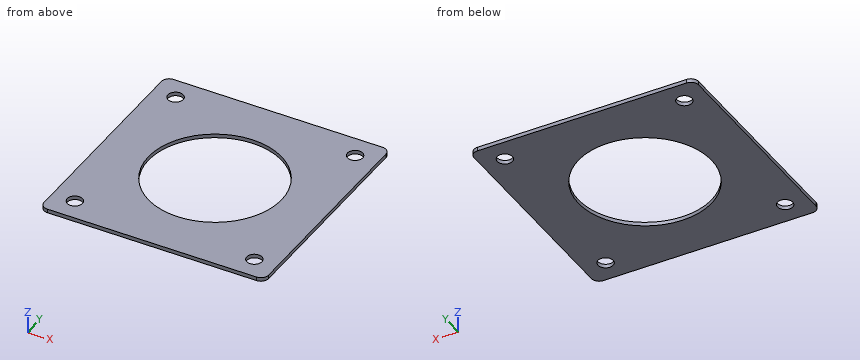
Autodesk Inventor part; units mm, degrees
ref_plane "YZ Plane" through (0, 0, 0) normal (1, 0, 0) x (0, 1, 0)
ref_plane "XZ Plane" through (0, 0, 0) normal (0, 1, 0) x (-1, 0, 0)
ref_plane "XY Plane" through (0, 0, 0) normal (0, 0, 1) x (1, 0, 0)
sketch "Sketch1" plane through (0, 0, 0) normal (0, 0, 1) x (1, 0, 0)
  line L0 (0, 0) -> (59, 0)
  line L1 (59, 0) -> (59, 59)
  line L2 (59, 59) -> (0, 59)
  line L3 (0, 59) -> (0, 0)
  dimension "d0" = 59
  dimension "d1" = 59
extrude "Extrusion1" add sketch "Sketch1" along normal blind 1
sketch "Sketch2" plane through (0, 0, 1) normal (0, 0, 1) x (1, 0, 0)
  circle A0 centre (29.5, 29.5) radius 17.5
  line L0 (59, 59) -> (0, 59)
  line L1 (0, 59) -> (0, 0)
  point P0 (29.5, 59)
  point P1 (0, 29.5)
  dimension "d4" = 35
extrude "Extrusion2" cut sketch "Sketch2" against normal through all
sketch "Sketch3" plane through (0, 0, 1) normal (0, 0, 1) x (1, 0, 0)
  line L0 (5.9, 5.9) -> (53.1, 5.9) construction
  line L1 (53.1, 5.9) -> (53.1, 53.1) construction
  line L2 (53.1, 53.1) -> (5.9, 53.1) construction
  line L3 (5.9, 53.1) -> (5.9, 5.9) construction
  line L4 (59, 59) -> (0, 59) construction
  line L5 (0, 59) -> (0, 0) construction
  circle A0 centre (5.9, 53.1) radius 2
  circle A1 centre (53.1, 53.1) radius 2
  circle A2 centre (53.1, 5.9) radius 2
  circle A3 centre (5.9, 5.9) radius 2
  point P0 (29.5, 53.1)
  point P1 (29.5, 59)
  point P2 (53.1, 29.5)
  point P3 (0, 29.5)
  dimension "d7" = 47.2
  dimension "d8" = 47.2
  dimension "d9" = 4
  dimension "d10" = 4
  dimension "d11" = 4
  dimension "d12" = 4
extrude "Extrusion3" cut sketch "Sketch3" against normal through all
fillet "Fillet1" radius 2 4 edges at (0, 59, 0.5) (59, 59, 0.5) (59, 0, 0.5) (0, 0, 0.5)
properties material "Aluminum 6061"
Source: CAD feature listing. Evaluate the final solid. Frame: model axes, mm. Coordinates: 2 decimals unless noted, no trailing zeros. Order: outer loops, then holes, each group sorted by start corner. A loop starts at its lowest first (then second) coordinate and runs counter-clockwise, first axis right, second up. Notation, with made-up numbers: M 19,-10 L 33,-10 A22 cw 33,1 Z; hole C 77.5,83.25 d11. An arc over 180 degrees is marked long. Write each question's results on one line, items separated by ' | '. Start each with the question number.
Item 1: First-contact query: pin 1 Ø2.5 at (x, y) = (53.1, 53.1) entering from +Z. Flat tip, straight axial feed; report the tip coordinate or a pass-through.
Item 2: Line query: probe 1 along Y at (x, z) = (53.1, 0.65); probe 2 along Y at (x, z) = (29.5, 0.35). Output: solid intervals per line, ascending.
Item 3: Cut plane A-A (y = 5.9). Return loops of the section in (x, z), and give its area (3 significant figures).
Item 4: Cut plane D-D (z = 0.4). Return loops of the section in (x, y), and give its area (3 significant figures).
Item 5: Cut plane B-B (x = 29.5). Return loops of the section in (y, z).
Checked values:
1) pin 1: passes through
2) probe 1: y = 0 to 3.9, 7.9 to 51.1, 55.1 to 59 | probe 2: y = 0 to 12, 47 to 59
3) outline: M 0,0 L 3.9,0 L 3.9,1 L 0,1 Z; M 7.9,0 L 51.1,0 L 51.1,1 L 7.9,1 Z; M 55.1,0 L 59,0 L 59,1 L 55.1,1 Z | area: 51.0 mm2
4) outline: M 0,2 A2 ccw 2,0 L 57,0 A2 ccw 59,2 L 59,57 A2 ccw 57,59 L 2,59 A2 ccw 0,57 Z; hole C 5.9,5.9 d4; hole C 5.9,53.1 d4; hole C 29.5,29.5 d35; hole C 53.1,5.9 d4; hole C 53.1,53.1 d4 | area: 2,470 mm2
5) outline: M 0,0 L 12,0 L 12,1 L 0,1 Z; M 47,0 L 59,0 L 59,1 L 47,1 Z
